```python
from build123d import *

# Parameters (mm, degrees)
BOSS_EXTRUDE1_DEPTH = 12
FILLET1_R           = 5
SKETCH5_W           = 13.25
SKETCH5_H           = 6
CUT_EXTRUDE3_DEPTH  = 35.785054262
SKETCH6_W           = 5
SKETCH6_H           = 2
BOSS_EXTRUDE2_DEPTH = 5
FILLET2_R           = 2.5
FILLET3_R           = 2.5
SKETCH3_R           = 1.65
CUT_EXTRUDE4_DEPTH  = 29.460498984
SKETCH8_R           = 0.75
CUT_EXTRUDE7_DEPTH  = 46.805137399
SKETCH9_R           = 0.75
CUT_EXTRUDE9_DEPTH  = 15.765865025


with BuildPart() as part:
    # Sketch2 → Boss-Extrude1 (new body)
    with BuildSketch(Plane.XY):
        with BuildLine():
            Line((-13.5, 0), (13.5, 0))
            ThreePointArc((13.5, 0), (21, -7.5), (13.5, -15))
            Line((13.5, -15), (-13.5, -15))
            ThreePointArc((-13.5, -15), (-21, -7.5), (-13.5, 0))
        make_face()
    extrude(amount=BOSS_EXTRUDE1_DEPTH)

    # Fillet1
    fillet1_edges = [part.edges().sort_by_distance(p)[0] for p in [
        (-21, -7.5, 12),
        (0, -15, 12),
        (21, -7.5, 12),
        (0, -15, 0),
        (-21, -7.5, 0),
        (0, 0, 0),
        (21, -7.5, 0),
        (0, 0, 12),
    ]]
    fillet(fillet1_edges, radius=FILLET1_R)

    # Sketch5 → Cut-Extrude3 (cut, through all)
    with BuildSketch(Plane(origin=(0, -25, 0), x_dir=(-1, 0, 0), z_dir=(0, -1, 0))):
        with Locations((14.375, -6)):
            Rectangle(SKETCH5_W, SKETCH5_H)
    extrude(amount=-CUT_EXTRUDE3_DEPTH, mode=Mode.SUBTRACT)

    # Sketch6 → Boss-Extrude2 (add)
    with BuildSketch(Plane(origin=(0, 0, 0), x_dir=(1, 0, 0), z_dir=(0, 1, 0))):
        with Locations((3, -6)):
            Rectangle(SKETCH6_W, SKETCH6_H)
    extrude(amount=BOSS_EXTRUDE2_DEPTH)

    # Fillet2
    fillet2_edges = [part.edges().sort_by_distance(p)[0] for p in [
        (5.5, 5, 6),
        (0.5, 5, 6),
    ]]
    fillet(fillet2_edges, radius=FILLET2_R - 0.0001)  # a hair under: the kernel refuses the full size

    # Fillet3
    fillet3_edges = [part.edges().sort_by_distance(p)[0] for p in [
        (0.5, 0, 6),
        (5.5, 0, 6),
    ]]
    fillet(fillet3_edges, radius=FILLET3_R)

    # Sketch3 → Cut-Extrude4 (cut, through all)
    with BuildSketch(Plane.XY.offset(12)):
        with Locations((-13.5, -7.5)):
            Circle(SKETCH3_R)
        with Locations((13.5, -7.5)):
            Circle(SKETCH3_R)
    extrude(amount=-CUT_EXTRUDE4_DEPTH, mode=Mode.SUBTRACT)

    # Sketch8 → Cut-Extrude7 (cut, through all)
    with BuildSketch(Plane(origin=(21, 0, 0), x_dir=(0, 0, -1), z_dir=(1, 0, 0))):
        with Locations((-6, -4)):
            Circle(SKETCH8_R)
    extrude(amount=-CUT_EXTRUDE7_DEPTH, mode=Mode.SUBTRACT)

    # Sketch9 → Cut-Extrude9 (cut, along a direction that is not the sketch's normal)
    with BuildSketch(Plane.ZY.offset(7.75)):
        with Locations((6, -11)):
            Circle(SKETCH9_R)
    extrude(amount=-CUT_EXTRUDE9_DEPTH, dir=(-0.9672796243913314, 0.25371268836493915, 0), mode=Mode.SUBTRACT)


solid = part.part
```
Input: part model. Units: mm. Frame: model coordinates. A direction names the side the tool comes from. Coordinates: 2 decimals unless noted, no trailing zeros. One line per item, written item: value.
(1) Pin query (flat end, axial travel): pin 1 (6 mm diameter, centred on y = 0.5, z = 2.5, fed in from -X); pin 2 (0.8 mm diameter, centred on y = -14.5, z = 6, fed in from -X); pin 3 (5.5 mm diameter, centred on x = 1, y = 1.5, fed in from +Z). Return the tip coordinate at first contact, or that it passes through.
Filled in:
pin 1: x = -18.47
pin 2: x = -7.75
pin 3: z = 10.31
(2) Line query: line 1 along X through (y, z) = (-6.5, 1); line 2 along Z through (x, y) = (-9, -2.25); line 3 along Y through (x, z) = (-13.5, 10.2). Output: solid intervals per line, ascending. Write a range as from..to.
Filled in:
line 1: -18.91..-14.81, -12.19..12.19, 14.81..18.91
line 2: 0.82..3, 9..11.18
line 3: -13.84..-9.15, -5.85..-1.16
(3) Section A-A (y = -7.5). Give the number of separate pieces and of enclosed holes in the cut face, and give its area (3 significant figures).
Filled in:
separate pieces: 4
enclosed holes: 0
area: 344 mm^2
(4) Pull-direction query (Y, two-part tool) for faces 4 (the flat face through (-5, 0, 6)), 5 (the flat face through (3, -15, 6)), 6 (the cylindrical face through (-11.976, -8.132, 1.521)); classes: +Y half, -Y half, draft (parallel to the pull), parting line (faces both ways), or undercut.
Filled in:
face 4: +Y half
face 5: -Y half
face 6: undercut
(5) Reachability of faces 1 (the cylindrical face through (6.561, -4.732, 6.163)), 2 (the flat face through (11, 0, 6)), 3 (the flat face through (-14.1, -9.2, 9)) from +Z, -Z, +X, -X, +Y, -Y: full face, straight path, thin tool, end or side. Return the list, or none.
Filled in:
face 1: +X, -X
face 2: +Z, -Z, +X, +Y
face 3: -X, +Y, -Y
